Build history of the part. All positions in model axes, mm. Face numbers are marked on the shaded views. A direction names the side the tool comes from. Round coordinates to 2 decimals unless told otherwise and drop trailing zeros. Write each loop counter-clockwise with the first axis right and the second up, starting at its lowest first coordinate (ties: lowest second). Pieces come first, ordered by that corner, then holes.
Item 1: Band-saw the part on A-A, the plane x = -40. Write the cut outline in (y, z).
Item 2: Band-saw the part on D-D, the plane x = 22.5. Write the cut outline in (y, z), then the cut area to 3 significant figures.
Item 3: Drop flat-ended pins along their axis: pin 1 Ø1 at (x, y) = (13, -17) entering from -Z; pin 2 Ø3 at (x, z) = (-15, 3) entering from +Y; pin 3 Ø3 at (x, y) = (-40, -15) entering from +Z. Give the stop position or say it passes through.
Item 4: Wall check: probe 1 along Y at (x, z) = (40, 3); probe 2 along X at (y, z) = (-14.25, 3.8); probe 3 along Z at (x, y) = (38, -9.75). Give the ranges that are in metal, low to high.
Item 5: 3-axis set-ups, long thin cutter, end or side, ignore diameter. For the marked faces 1, 2 and 3: which of +Z, -Z, +X, -X, +Y, -Y reach the whole face in a straight line?
Item 6: Band-saw the part on C-C, the plane y = -15. Write the cut outline in (x, z).
Item 7: Band-saw the part on B-B, the plane y = -5. Write the cut outline in (x, z).
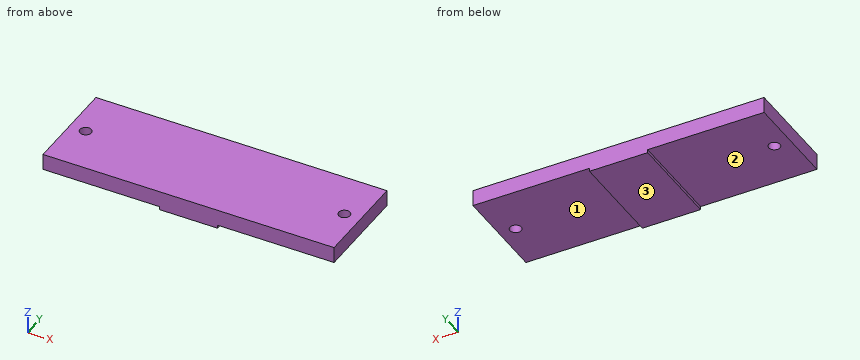
```python
from build123d import *

# Parameters (mm, degrees)
SKETCH1_W           = 90
SKETCH1_H           = 30
BOSS_EXTRUDE1_DEPTH = 5
SKETCH2_R           = 1.75
CUT_EXTRUDE1_DEPTH  = 55.313902456
SKETCH3_W           = 18
SKETCH3_H           = 30
BOSS_EXTRUDE2_DEPTH = 1


with BuildPart() as part:
    # Sketch1 → Boss-Extrude1 (new body)
    with BuildSketch(Plane.XY):
        with Locations((0, -15)):
            Rectangle(SKETCH1_W, SKETCH1_H)
    extrude(amount=BOSS_EXTRUDE1_DEPTH)

    # Sketch2 → Cut-Extrude1 (cut, through all)
    with BuildSketch(Plane.XY.offset(5)):
        with Locations((40, -15)):
            Circle(SKETCH2_R)
        with Locations((-40, -15)):
            Circle(SKETCH2_R)
    extrude(amount=-CUT_EXTRUDE1_DEPTH, mode=Mode.SUBTRACT)

    # Sketch3 → Boss-Extrude2 (add)
    with BuildSketch(Plane(origin=(0, 0, 0), x_dir=(-1, 0, 0), z_dir=(0, 0, -1))):
        with Locations((0, -15)):
            Rectangle(SKETCH3_W, SKETCH3_H)
    extrude(amount=BOSS_EXTRUDE2_DEPTH)


solid = part.part
```
Results:
1. outline: (-30, 0) - (-16.75, 0) - (-16.75, 5) - (-30, 5) - close; (-13.25, 0) - (0, 0) - (0, 5) - (-13.25, 5) - close
2. outline: (-30, 0) - (0, 0) - (0, 5) - (-30, 5) - close
2. area: 150 mm2
3. pin 1: stops at z = 0
3. pin 2: stops at y = 0
3. pin 3: passes through
4. probe 1: y = -30 to -16.75, -13.25 to 0
4. probe 2: x = -45 to -41.58, -38.42 to 38.42, 41.58 to 45
4. probe 3: z = 0 to 5
5. face 1: -Z, +X, +Y, -Y
5. face 2: -Z, -X, +Y, -Y
5. face 3: -Z, +X, -X, +Y, -Y
6. outline: (-45, 0) - (-41.75, 0) - (-41.75, 5) - (-45, 5) - close; (-38.25, 0) - (-9, 0) - (-9, -1) - (9, -1) - (9, 0) - (38.25, 0) - (38.25, 5) - (-38.25, 5) - close; (41.75, 0) - (45, 0) - (45, 5) - (41.75, 5) - close
7. outline: (-45, 0) - (-9, 0) - (-9, -1) - (9, -1) - (9, 0) - (45, 0) - (45, 5) - (-45, 5) - close
